Could you check a few things on this model? Use its own coordinates, in mm. Face numbers are marked on the shaded views. Coordinates: 2 decimals unless noted, no trailing zeros. Loops run counter-clockwise (first coordinate to the right, second up) from the corner with the lowest first, then second, coordinate; pieces in that order, holes last. Notation, with made-up numbers: (-1.75, 2.5) -> (55.25, 2.5) arc R22 cw to (55.25, 30.5) -> close; hole circle Ø2 at (13, 0.5). An arc over 180 degrees is marked (long way). One line per question, with ' | ' between items. Start each with the question number.
(1) If we mould it in two halves opening along X, with no side actions, what happens to the marked faces 1, 2 and 3? For each: pulls with the +X half, pulls with the -X half, needs draft (parallel to the pull), parting line crosses it, or undercut.
(2) Suppose I cut it at C-C (y = -15.5). Please give me the cut outline in (x, z), plus the area to 3 significant figures.
(3) Suppose I cut it at A-A (z = 0). Please give me the cut outline in (x, y), plus the area to 3 significant figures.
(4) If I drill on line 1 along Z through (x, y) = (0, -11); line 2 along Z through (x, y) = (7.5, -16); line 3 along X through (y, z) = (-21.25, -23), over which ranges is the centre line in solid material (lowest first)?
(5) I'm going to push a flat-ended pin straight in: pin 1 Ø15 at (x, z) = (0, 24.97) entering from -Y. Where does the tip first touch, or does it pass through?
(6) Suppose I cut it at D-D (z = -21.5). Please give me the cut outline in (x, y), plus the area to 3 significant figures.
(7) Suppose I cut it at B-B (x = 0). Please give me the cut outline in (y, z).
```python
from build123d import *

# Parameters (mm, degrees)
F2_W        = 25.9886477143
F2_H        = 80.8860212564
F2_R        = 10.2254684018
F2_R_2      = 9.290469056
F3_DEPTH    = 25.4
F4_D        = 25.4
F5_T1_DEPTH = 106.2860212564


# Not quite as in the source:
# - a fillet or chamfer that OpenCascade refuses, or shapes differently, is made with other operations: its cross-section is extruded or revolved along the edge and cut away or added
# - a feature names something its author has since deleted; it is built from what else it names


with BuildPart() as f3:
    # F2 (on face) → F3 (new body)
    with BuildSketch(Plane.XZ):
        Rectangle(F2_W, F2_H)
        with Locations((0, -25.5506392568)):
            Circle(F2_R, mode=Mode.SUBTRACT)
        with Locations((0, 24.9666236341)):
            Circle(F2_R_2, mode=Mode.SUBTRACT)
    extrude(amount=F3_DEPTH)

    # F4 (through all)
    with Locations(Plane(origin=(0, 0, 0), x_dir=(1, 0, 0), z_dir=(0, 1, 0))):
        with Locations((0, 0)):
            Hole(F4_D / 2)

    # F5: fillet of radius 5.08 on 3 edges, made by hand

    # F5_s2 → F5_t1 (cut)
    with BuildSketch(Plane.XY.offset(-53.1430106282)):
        with BuildLine():
            ThreePointArc((7.9143238571, 0), (11.5064263056, -1.4878975516), (12.9943238571, -5.08))
            Line((12.9943238571, -5.08), (12.9943238571, 0))
            Line((12.9943238571, 0), (7.9143238571, 0))
        make_face()
        with BuildLine():
            ThreePointArc((7.9143238571, -25.4), (11.5064263056, -23.9121024484), (12.9943238571, -20.32))
            Line((12.9943238571, -20.32), (12.9943238571, -25.4))
            Line((12.9943238571, -25.4), (7.9143238571, -25.4))
        make_face()
    extrude(amount=F5_T1_DEPTH, mode=Mode.SUBTRACT)

    # F5_s3 → F5_t4 (revolve, cut)
    with BuildSketch(Plane.XY):
        with BuildLine():
            ThreePointArc((17.78, 0), (14.1878975516, -1.4878975516), (12.7, -5.08))
            Line((12.7, -5.08), (12.7, 0))
            Line((12.7, 0), (17.78, 0))
        make_face()
    revolve(axis=Axis((0, 0, 0), (0, 1, 0)), mode=Mode.SUBTRACT)


solid = f3.part
```
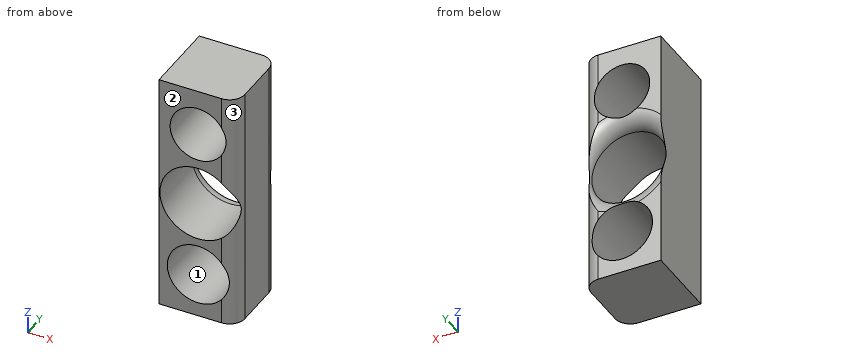
Checks:
1) face 1: undercut | face 2: needs draft | face 3: pulls with the +X half
2) outline: (-12.99, -40.44) -> (12.99, -40.44) -> (12.99, 40.44) -> (-12.99, 40.44) -> close; hole circle Ø25.4 at (0, 0); hole circle Ø20.45 at (0, -25.55); hole circle Ø18.58 at (0, 24.97) | area: 996 mm^2
3) outline: (-12.99, -25.4) -> (-12.7, -25.4) -> (-12.7, -5.08) arc R5.08 ccw to (-12.99, -3.38) -> close; (12.7, -22.02) arc R5.08 ccw to (12.99, -20.32) -> (12.99, -5.08) arc R5.08 ccw to (12.85, -3.87) arc R5.08 ccw to (12.7, -5.08) -> close | area: 11.4 mm^2
4) line 1: z = -40.44 to -35.78, -15.33 to -12.7, 12.7 to 15.68, 34.26 to 40.44 | line 2: z = -40.44 to -32.5, -18.6 to -10.25, 10.25 to 19.48, 30.45 to 40.44 | line 3: x = -12.99 to -9.9, 9.9 to 12.91
5) pin 1: passes through
6) outline: (-12.99, -25.4) -> (-9.39, -25.4) -> (-9.39, 0) -> (-12.99, 0) -> close; (9.39, -25.18) arc R5.08 ccw to (12.99, -20.32) -> (12.99, -5.08) arc R5.08 ccw to (9.39, -0.22) -> close | area: 172 mm^2
7) outline: (-25.4, -40.44) -> (0, -40.44) -> (0, -35.78) -> (-25.4, -35.78) -> close; (-25.4, -15.33) -> (-0.63, -15.33) arc R5.08 ccw to (-5.08, -12.7) -> (-25.4, -12.7) -> close; (-25.4, 12.7) -> (-5.08, 12.7) arc R5.08 ccw to (-0.46, 15.68) -> (-25.4, 15.68) -> close; (-25.4, 34.26) -> (0, 34.26) -> (0, 40.44) -> (-25.4, 40.44) -> close
